Could you check a few things on this drawing? It's one solid part, dimensions in mm from its lowest x, y, z. A direction names the side the tool comes from. Give positions to 0.01 mm unless a question says otherwise; leave off trailing zeros. Loops run counter-clockwise (first coordinate to the right, second up) from the corner with the lowest first, then second, coordinate; pieces in that order, holes last. Notation, with made-up numbers: M 59,33 L 102,33 A18 cw 102,39 Z; hole C 74,54 d3. An arc over 180 degrees is marked long. Answer in a Markdown table with one row per item. Add a question column.
1. If we section it at A-A on x = 16.5: List the corners of the cut face in (y, z) for me.
2. If we section it at D-D on y = 23.5: List the corners of the cut face in (x, z) for me, then the cut area to 3 significant figures.
3. Which directions (+Z, -Z, +X, -X, +Y, -Y) give clear straight access to the entire face, cutting with the end or side of a thin tool? Please do the marked faces 1, 2 and 3.
4. If we section it at B-B on z = 20.75: List the corners of the cut face in (x, y) for me, then the cut area to 3 significant figures.
5. I'm going to push flat-ended pins straight in: pin 1 Ø3 at (x, z) = (38.5, 24) entering from +Y; pin 2 Ø4 at (x, z) = (5, 25.5) entering from -Y; pin 3 Ø20.5 at (x, y) = (11, 26) entering from +Z. Where does each tip first touch, or does it pass through?
6. Thinking about a two-plate mould opening in Y: for the marked faces 4, 5, 6 and 7, which applies, released by +Y, released by -Y, zero draft, split by the parting line, or undercut?
7. If we section it at C-C on z = 2.5: List the corners of the cut face in (x, y) for me.
8. I need wall thicknesses on line 1 along Z through (x, y) = (5, 4); line 2 along Y through (x, z) = (26, 3.5); line 3 along X through (y, z) = (5.5, 25.5) (3 decimals). Which ranges of each line are inside material? Lowest first, please. Write a range as from..to.
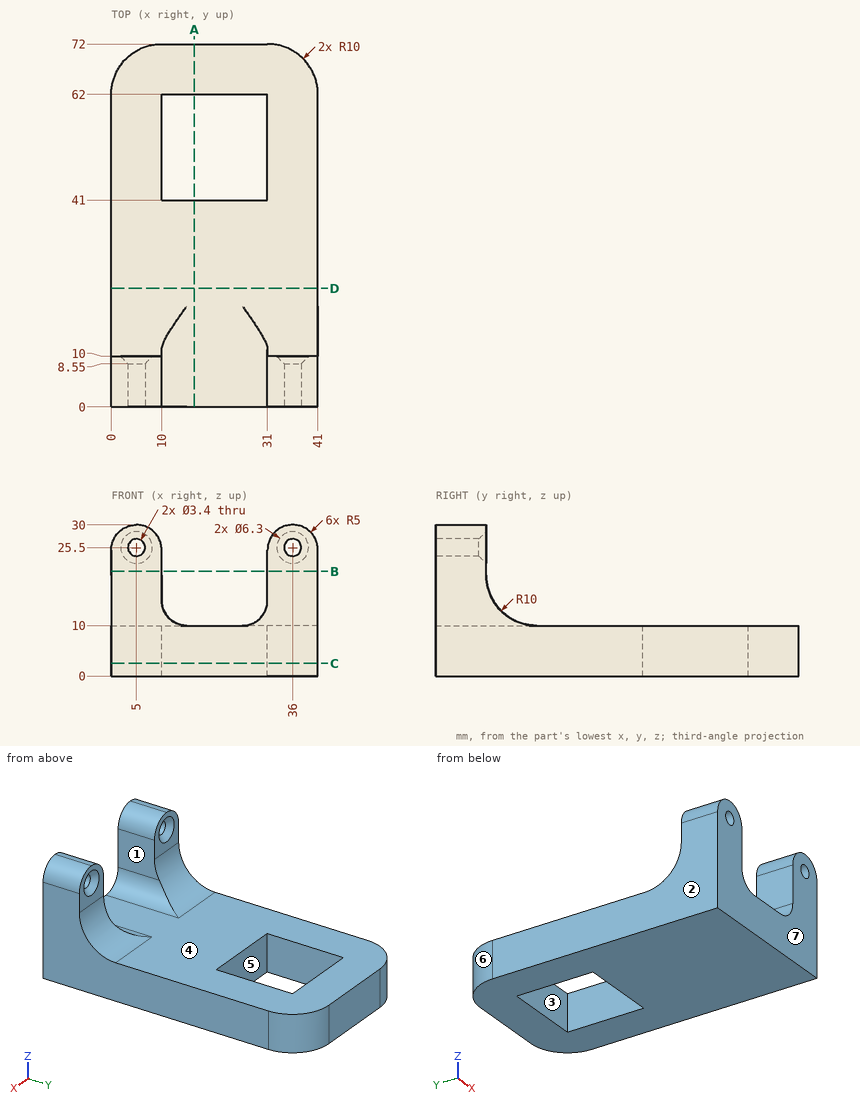
Results:
| question | item | result |
|---|---|---|
| 1 | outline | M 0,0 L 41,0 L 41,10 L 0,10 Z; M 62,0 L 72,0 L 72,10 L 62,10 Z |
| 2 | outline | M 0,0 L 41,0 L 41,10 L 0,10 Z |
| 2 | area | 410 mm2 |
| 3 | face 1 | +Z, +Y, -Y |
| 3 | face 2 | +Z, -Z, -X, +Y, -Y |
| 3 | face 3 | +Z, -Z |
| 4 | outline | M 0,0 L 10,0 L 10,10 L 0,10 Z; M 31,0 L 41,0 L 41,10 L 31,10 Z |
| 4 | area | 200 mm2 |
| 5 | pin 1 | y = 10 |
| 5 | pin 2 | y = 0 |
| 5 | pin 3 | z = 10.95 |
| 6 | face 4 | zero draft |
| 6 | face 5 | undercut |
| 6 | face 6 | released by +Y |
| 6 | face 7 | released by -Y |
| 7 | outline | M 0,0 L 41,0 L 41,62 A10 ccw 31,72 L 10,72 A10 ccw 0,62 Z; hole M 10,41 L 31,41 L 31,62 L 10,62 Z |
| 8 | line 1 | 0..23.8, 27.2..30 |
| 8 | line 2 | 0..41, 62..72 |
| 8 | line 3 | 0.025..3.3, 6.7..9.975, 31.025..34.3, 37.7..40.975 |
